Autodesk Inventor part; units mm, degrees
ref_plane "YZ Plane" through (0, 0, 0) normal (1, 0, 0) x (0, 1, 0)
ref_plane "XZ Plane" through (0, 0, 0) normal (0, 1, 0) x (-1, 0, 0)
ref_plane "XY Plane" through (0, 0, 0) normal (0, 0, 1) x (1, 0, 0)
sketch "Sketch1" plane through (0, 0, 0) normal (0, 1, 0) x (-1, 0, 0)
  arc A0 (17.4776, 61.9438) -> (-14.1045, 61.9438) centre (1.6865, 55.6475) ccw
  arc A1 (-14.1045, -58.6488) -> (17.4776, -58.6488) centre (1.6865, -52.3525) ccw
  line L0 (36.0552, 15.3512) -> (17.4776, 61.9438)
  line L1 (-14.1045, 61.9438) -> (-32.6822, 15.3512)
  line L2 (-32.6822, -12.0562) -> (-14.1045, -58.6488)
  line L3 (17.4776, -58.6488) -> (36.0552, -12.0562)
  arc A2 (-32.6822, 15.3512) -> (-32.6822, -12.0562) centre (1.6865, 1.6475) ccw
  arc A3 (36.0552, -12.0562) -> (36.0552, 15.3512) centre (1.6865, 1.6475) ccw
  circle A4 centre (1.6865, 55.6475) radius 6.5
  circle A5 centre (1.6865, -52.3525) radius 6.5
  circle A6 centre (1.6865, 1.6475) radius 26
  dimension "d11" = 13
  dimension "d12" = 13
  dimension "d13" = 52
extrude "Extrusion1" add sketch "Sketch1" along normal blind 14
sketch "Sketch2" plane through (0, 14, 0) normal (0, 1, 0) x (1, 0, 0)
  circle A0 centre (-1.6865, -1.6475) radius 26
  circle A1 centre (-1.6865, -1.6475) radius 32
  point P0 (0, 0)
  dimension "d16" = 64
extrude "Extrusion2" add sketch "Sketch2" along normal blind 2
properties part number "00.32.011 \"Flange\""
Work out the finished part from the listing and answer in its coordinate system (mm). A direction names the side the tool comes from. Give positions to 0.01 mm unless a question says otherwise; leave off trailing zeros. Write each loop counter-clockwise with the first axis right and the second up, starting at its lowest first coordinate (ties: lowest second). Pieces come first, ordered by that corner, then holes. Notation, with made-up numbers: (36.25, 25) - (47.25, 25) arc R21 cw to (47.25, 38) - close; hole circle Ø4 at (16, 57.5). An arc over 180 degrees is marked (long way). One line per item, written item: value. Start each with the question number.
1. Find section C-C (y = 5.5). Write down the section's boundary in (x, z).
2. Given pin 1 (6 mm diameter, centred on y = 10.5, z = 46.5, fed in from +X); pin 2 (3 mm diameter, centred on y = 13, z = -12, fed in from +X); pin 3 (21 mm diameter, centred on x = -1.69, z = -52.35, fed in from +Y), each flat-ended and moving along its own axis, determine where each tip first touches the part or whether it passes through.
3. Find section D-D (z = 51). Write down the section's boundary in (x, y), then the cut area to 3 significant figures.
4. Find section A-A (z = -6). Write down the section's boundary in (x, y), then the cut area to 3 significant figures.
5. For a pull along Z with two mould halves and no side action, classify faces 3 (the flat face through (-26, 0, -13)), 4 (the cylindrical face through (35.313, 6.902, 1.451)), 5 (the cylindrical face through (-0.277, 6.902, -46.007)) as +Z half, -Z half, draft (parallel to the pull), parting line (faces both ways), or undercut.
6. Consider probe 1 along Z at (x, y) = (-9, 6.5); probe 2 along Y at (x, z) = (5.5, 65); probe 3 along Z at (x, y) = (-0.5, 8.75). Determine where each line is inside the solid, lowest interval first.
7. For faces 1 (the cylindrical face through (-5.852, 14.986, 33.375)), 2 (the flat face through (-26.896, 6.902, 38.321)), determine the directions among +Z, -Z, +X, -X, +Y, -Y from which every point of the face is accessible in a straight line to the end or side of a thin tool.
Geometry results:
1. outline: (-36.06, -12.06) - (-17.48, -58.65) arc R17 ccw to (14.1, -58.65) - (32.68, -12.06) arc R37 ccw to (32.68, 15.35) - (14.1, 61.94) arc R17 ccw to (-17.48, 61.94) - (-36.06, 15.35) arc R37 ccw to start; hole circle Ø52 at (-1.69, 1.65); hole circle Ø13 at (-1.69, -52.35); hole circle Ø13 at (-1.69, 55.65)
2. pin 1: x = 21.46
2. pin 2: x = 33.26
2. pin 3: y = 14
3. outline: (-21.84, 0) - (-6.23, 0) - (-6.23, 14) - (-21.84, 14) - close; (2.86, 0) - (18.47, 0) - (18.47, 14) - (2.86, 14) - close
3. area: 437 mm2
4. outline: (-37.89, 0) - (-26.54, 0) - (-26.54, 16) - (-32.76, 16) - (-32.76, 14) - (-37.89, 14) - close; (23.16, 0) - (34.51, 0) - (34.51, 14) - (29.39, 14) - (29.39, 16) - (23.16, 16) - close
4. area: 343 mm2
5. face 3: draft
5. face 4: parting line
5. face 5: undercut
6. probe 1: -67.7 to -23.3, 26.6 to 70.99
6. probe 2: 0 to 14
6. probe 3: -69.31 to -58.74, -45.96 to -24.33, 27.62 to 49.26, 62.04 to 72.61
7. face 1: +Y
7. face 2: +Z, -X, +Y, -Y
